Source: CAD feature listing. Evaluate the final solid. Frame: model axes, mm. Coordinates: 2 decimals unless noted, no trailing zeros. Write each loop counter-clockwise with the first axis right and the second up, starting at its lowest first coordinate (ties: lowest second). Pieces come first, ordered by that corner, then holes. Notation, with made-up numbers: (48, 88.25) - (59, 88.25) arc R20 ccw to (59, 99.25) - close; hole circle Ø2 at (-25.5, 4). An arc over 180 degrees is marked (long way). One line per question, with ' | ' between items. Start each with the question number.
Q1. Cut plane A-A, the plane z = 1.05. Return loops of the section in (x, y), plus the area to 3 significant figures.
Q2. Contact query for flat-ended pins moving along their axis: P1, Ø1, axis at y = 23, z = 0.5, coming from the -X side; P2, Ø0.6, axis at y = 64.5, z = 1, coming from the +X side. Output: stop coordinate, or through.
Q3. Cut plane B-B, the plane y = 64.5. Return loops of the section in (x, z).
Q4. Cut plane C-C, the plane x = -7. Return loops of the section in (y, z).
Q5. Line query: line 1 (Y direction, x = 12.5, z = 1.4); line 2 (X direction, y = 55, z = 0.9); line 3 (X direction, y = 27, z = 0.45). Output: solid intervals per line, ascending.
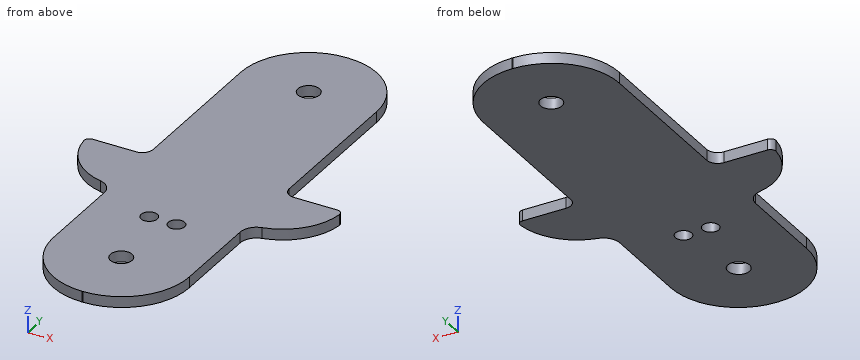
```python
from build123d import *

# Parameters (mm, degrees)
SKETCH1_R           = 2
SKETCH1_R_2         = 1.5
BOSS_EXTRUDE1_DEPTH = 2


with BuildPart() as part:
    # Sketch1 → Boss-Extrude1 (new body)
    with BuildSketch(Plane.XY):
        with BuildLine():
            Line((12.4, 0), (12.6, 0))
            ThreePointArc((12.6, 0), (21.368124087, 3.631875913), (25, 12.4))
            Line((25, 12.4), (25, 28.774148297))
            ThreePointArc((25, 28.774148297), (25.663151139, 30.655407822), (27.359424934, 31.704961083))
            ThreePointArc((27.359424934, 31.704961083), (33.251440199, 35.15061323), (35.99503719, 41.400496281))
            ThreePointArc((35.99503719, 41.400496281), (35.741452534, 42.171005321), (35, 42.5))
            Line((35, 42.5), (27, 42.5))
            ThreePointArc((27, 42.5), (25.585786438, 43.085786438), (25, 44.5))
            Line((25, 44.5), (25, 72.6))
            ThreePointArc((25, 72.6), (21.368124087, 81.368124087), (12.6, 85))
            Line((12.6, 85), (12.4, 85))
            ThreePointArc((12.4, 85), (3.631875913, 81.368124087), (0, 72.6))
            Line((0, 72.6), (0, 44.5))
            ThreePointArc((0, 44.5), (-0.585786438, 43.085786438), (-2, 42.5))
            Line((-2, 42.5), (-10, 42.5))
            ThreePointArc((-10, 42.5), (-10.741452534, 42.171005321), (-10.99503719, 41.400496281))
            ThreePointArc((-10.99503719, 41.400496281), (-8.251440199, 35.15061323), (-2.359424934, 31.704961083))
            ThreePointArc((-2.359424934, 31.704961083), (-0.663151139, 30.655407822), (0, 28.774148297))
            Line((0, 28.774148297), (0, 12.4))
            ThreePointArc((0, 12.4), (3.631875913, 3.631875913), (12.4, 0))
        make_face()
        with Locations((12.5, 72.6)):
            Circle(SKETCH1_R, mode=Mode.SUBTRACT)
        with Locations((12.5, 12.4)):
            Circle(SKETCH1_R, mode=Mode.SUBTRACT)
        with Locations((10, 25.767183826)):
            Circle(SKETCH1_R_2, mode=Mode.SUBTRACT)
        with Locations((15, 25.767183826)):
            Circle(SKETCH1_R_2, mode=Mode.SUBTRACT)
    extrude(amount=BOSS_EXTRUDE1_DEPTH)


solid = part.part
```
Reply:
1) outline: (-11, 41.4) arc R11.05 ccw to (-2.36, 31.7) arc R3 cw to (0, 28.77) - (0, 12.4) arc R12.4 ccw to (12.4, 0) - (12.6, 0) arc R12.4 ccw to (25, 12.4) - (25, 28.77) arc R3 cw to (27.36, 31.7) arc R11.05 ccw to (36, 41.4) arc R1 ccw to (35, 42.5) - (27, 42.5) arc R2 cw to (25, 44.5) - (25, 72.6) arc R12.4 ccw to (12.6, 85) - (12.4, 85) arc R12.4 ccw to (0, 72.6) - (0, 44.5) arc R2 cw to (-2, 42.5) - (-10, 42.5) arc R1 ccw to start; hole circle Ø3 at (10, 25.77); hole circle Ø4 at (12.5, 12.4); hole circle Ø4 at (12.5, 72.6); hole circle Ø3 at (15, 25.77) | area: 2,150 mm^2
2) P1: stops at x = 0 | P2: stops at x = 25
3) outline: (0, 0) - (25, 0) - (25, 2) - (0, 2) - close
4) outline: (33.95, 0) - (42.5, 0) - (42.5, 2) - (33.95, 2) - close
5) line 1: y = 0 to 10.4, 14.4 to 70.6, 74.6 to 85 | line 2: x = 0 to 25 | line 3: x = 0 to 9.15, 10.85 to 14.15, 15.85 to 25
